```python
from build123d import *

# Parameters (mm, degrees)
SKETCH_1_R      = 2
SKETCH_1_R_2    = 1
EXTRUDE_1_DEPTH = 70
SKETCH_2_W      = 0.5
SKETCH_2_H      = 3
SKETCH_3_W      = 0.5
SKETCH_3_H      = 45


with BuildPart() as part:
    # Эскиз1 → Бобышка-Вытянуть1 (new body)
    with BuildSketch(Plane(origin=(0, 0, 0), x_dir=(1, 0, 0), z_dir=(0, 1, 0))):
        Circle(SKETCH_1_R)
        Circle(SKETCH_1_R_2, mode=Mode.SUBTRACT)
    extrude(amount=EXTRUDE_1_DEPTH)

    # Эскиз2 → Вырез-Повернуть1 (revolve, cut)
    with BuildSketch(Plane.XY):
        with Locations((1.75, 68.5)):
            Rectangle(SKETCH_2_W, SKETCH_2_H)
        with Locations((1.75, 61.5)):
            Rectangle(SKETCH_2_W, SKETCH_2_H)
    revolve(axis=Axis((0, 70, 0), (0, -1, 0)), mode=Mode.SUBTRACT)

    # Эскиз3 → Вырез-Повернуть2 (revolve, cut)
    with BuildSketch(Plane.XY):
        with Locations((1.75, 22.5)):
            Rectangle(SKETCH_3_W, SKETCH_3_H)
    revolve(axis=Axis((0, 0, 0), (0, 1, 0)), mode=Mode.SUBTRACT)


solid = part.part
```
Model file for the job. Use its own axes, mm. A direction names the side the tool comes from. Give positions to 0.01 mm unless a question says otherwise; leave off trailing zeros. Loops run counter-clockwise (first coordinate to the right, second up) from the corner with the lowest first, then second, coordinate; pieces in that order, holes last. Notation, with made-up numbers: (-25, 58.25) - (-10, 58.25) arc R9 ccw to (-10, 73.25) - close; hole circle Ø1 at (10, 44.25). An arc over 180 degrees is marked (long way). One line per item, written item: value. Start each with the question number.
1. Slice it at A-A (z = 0). List the corners of the cut face in (x, y).
2. Pull direction Z, two halves, no side cores. Call faces 1 (the cylindrical face through (0, 35, 1)), 2 (the cylindrical face through (0, 52, 2)): pulls with the +Z half, pulls with the -Z half, needs draft (parallel to the pull), parting line crosses it, or undercut.
3. Slice it at B-B (x = 0.25). List the corners of the cut face in (y, z).
4. Which spindle directions (+Z, -Z, +X, -X, +Y, -Y) get a long thin tool onto all of the face, cutting with end or side? Do faces 3 (the cylindrical face through (-1.5, 22.82, -0.07)), 4 (the cylindrical face through (-1.5, 61.52, 0.07)), 5 (the cylindrical face through (-1.5, 68.52, 0.07)). Say none if no direction does.
5. Slice it at C-C (y = 31.5). List the corners of the cut face in (x, z).
6. Probe L1, parallel to X at y = 19.5, z = 0; L2, parallel to Y at x = 0.75, z = 1.5. List the from-to ranges inside material, lowest first. Write a range as from..to.
7. Pin check, flat tips, straight feed: pin 1 (2 mm diameter, centred on x = 0.5, y = 39.5, fed in from -Z); pin 2 (1 mm diameter, centred on y = 9.5, z = -1, fed in from -X). Stop position of each tip, or through.
Solution:
1. outline: (-2, 45) - (-1.5, 45) - (-1.5, 0) - (-1, 0) - (-1, 70) - (-1.5, 70) - (-1.5, 67) - (-2, 67) - (-2, 63) - (-1.5, 63) - (-1.5, 60) - (-2, 60) - close; (1, 0) - (1.5, 0) - (1.5, 45) - (2, 45) - (2, 60) - (1.5, 60) - (1.5, 63) - (2, 63) - (2, 67) - (1.5, 67) - (1.5, 70) - (1, 70) - close
2. face 1: undercut
2. face 2: parting line crosses it
3. outline: (0, -1.48) - (45, -1.48) - (45, -1.98) - (60, -1.98) - (60, -1.48) - (63, -1.48) - (63, -1.98) - (67, -1.98) - (67, -1.48) - (70, -1.48) - (70, -0.97) - (0, -0.97) - close; (0, 0.97) - (70, 0.97) - (70, 1.48) - (67, 1.48) - (67, 1.98) - (63, 1.98) - (63, 1.48) - (60, 1.48) - (60, 1.98) - (45, 1.98) - (45, 1.48) - (0, 1.48) - close
4. face 3: -Y
4. face 4: none
4. face 5: +Y
5. outline: circle Ø3 at (0, 0); hole circle Ø2 at (0, 0)
6. L1: x = -1.5..-1, 1..1.5
6. L2: y = 45..60, 63..67
7. pin 1: stops at z = -1.5
7. pin 2: stops at x = -1.41
